Autodesk Inventor part; units mm, degrees
ref_plane "YZ Plane" through (0, 0, 0) normal (1, 0, 0) x (0, 1, 0)
ref_plane "XZ Plane" through (0, 0, 0) normal (0, 1, 0) x (-1, 0, 0)
ref_plane "XY Plane" through (0, 0, 0) normal (0, 0, 1) x (1, 0, 0)
sketch "Sketch1" plane through (0, 0, 0) normal (0, 1, 0) x (-1, 0, 0)
  arc A0 (41.4246, 2.5) -> (41.4246, -2.5) centre (0, 0) ccw construction
  line L0 (0, -41.5) -> (0, 41.5)
  line L1 (0, 0) -> (41.5, 0) construction
  line L2 (41.4246, 2.5) -> (43.7, 2.5)
  line L3 (43.7, 2.5) -> (43.7, -2.5)
  line L4 (43.7, -2.5) -> (41.4246, -2.5)
  line L5 (39.3, 2.5) -> (43.7, -2.5) construction
  line L6 (43.7, 2.5) -> (39.3, -2.5) construction
  arc A1 (0, -41.5) -> (41.4246, -2.5) centre (0, 0) ccw
  arc A2 (41.4246, 2.5) -> (0, 41.5) centre (0, 0) ccw
  line L7 (41.4246, -2.5) -> (41.4246, 2.5) construction
  line L8 (2, 39.4493) -> (2, -39.4493)
  arc A3 (2, -39.4493) -> (39.4968, -0.5) centre (0, 0) ccw
  line L9 (39.4968, -0.5) -> (41.7, -0.5)
  line L10 (41.7, -0.5) -> (41.7, 0.5)
  line L11 (41.7, 0.5) -> (39.4968, 0.5)
  arc A4 (39.4968, 0.5) -> (2, 39.4493) centre (0, 0) ccw
  dimension "d0" = 83
  dimension "d1" = 83
  dimension "d2" = 5
  dimension "d4" = 2.2
  dimension "d5" = 41.5
  dimension "d6" = 2
extrude "Extrusion1" add sketch "Sketch1" against normal blind 2 contours L0 A2 L2 L3 L4 A1 | A4 L11 L10 L9 A3 L8
extrude "Extrusion2" add sketch "Sketch1" along normal blind 173
sketch "Sketch2" plane through (0, -2, 41.5) normal (1, 0, 0) x (0, 0, -1)
  circle A0 centre (12, 12) radius 4.5
  line L0 (83, 0) -> (0, 0)
  line L1 (0, 0) -> (0, 175)
  point P0 (41.5, 2)
  dimension "d11" = 9
  dimension "d12" = 12
  dimension "d13" = 12
extrude "Extrusion3" cut sketch "Sketch2" against normal blind 10
properties part number "_3DPrint"
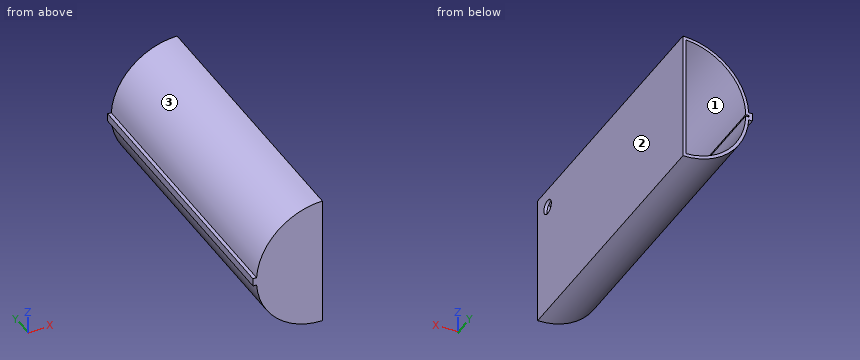
The listing builds one solid part. Answer for the finished solid, in the listing's coordinates (mm). Face numbers are marked on the shaded views. Give positions to 0.01 mm unless a question says otherwise; leave off trailing zeros. Order: outer loops, then holes, each group sorted by start corner. A loop starts at its lowest first (then second) coordinate and runs counter-clockwise, first axis right, second up. Notation, with made-up numbers: (88.25, -33.75) -> (119.25, -33.75) arc R24 cw to (119.25, -10.75) -> close; hole circle Ø2 at (-9, 47). An arc over 180 degrees is marked (long way). Write each question's results on one line, items separated by ' | '.
Q1. Determine the mould class of the marked faces 1, 2 and 3 for opening direction Z: pulls with the +Z half, pulls with the -Z half, needs draft (parallel to the pull), parting line crosses it, or undercut.
Checked values:
face 1: undercut | face 2: needs draft | face 3: pulls with the +Z half
Q2. The part is cut by section A-A, the plane y = 153. Give the vertices of the cut face in (x, z).
Checked values:
outline: (-43.7, -2.5) -> (-41.42, -2.5) arc R41.5 ccw to (0, -41.5) -> (0, 41.5) arc R41.5 ccw to (-41.42, 2.5) -> (-43.7, 2.5) -> close; hole (-41.7, -0.5) -> (-39.5, -0.5) arc R39.5 ccw to (-2, -39.45) -> (-2, 39.45) arc R39.5 ccw to (-39.5, 0.5) -> (-41.7, 0.5) -> close
Q3. The part is cut by section D-D, the plane x = -26.5. Give the vertices of the cut face in (y, z), and give its area (3 significant figures).
Checked values:
outline: (-2, -31.94) -> (173, -31.94) -> (173, -29.29) -> (0, -29.29) -> (0, 29.29) -> (173, 29.29) -> (173, 31.94) -> (-2, 31.94) -> close | area: 1,040 mm^2
Q4. Straight lines are drawn through the part: probe 1 along Y at (x, z) = (-0.55, 29.5); probe 2 along X at (y, z) = (132, -2); probe 3 along X at (y, z) = (139.5, -1.5). For each, find the intervals that lie inside material, in ascending order. Write a range as from..to.
Checked values:
probe 1: y = -2..5.5, 14.5..173 | probe 2: x = -43.7..-39.45, -2..0 | probe 3: x = -43.7..-39.47, -2..0
Q5. Each of these flat-tipped pins is pushed along its axis until it touches: P1, Ø12, axis at x = -14.5, y = 77.5, coming from the +Z side; P2, Ø10, axis at x = -8, y = 125, coming from the -Z side; P3, Ø3, axis at x = -8.5, y = 152.5, coming from the -Z side; P4, Ø10, axis at x = -32.5, z = 18.5, coming from the +Y side. Where does it stop, or does it pass through?
Checked values:
P1: stops at z = 40.62 | P2: stops at z = -41.39 | P3: stops at z = -40.91 | P4: stops at y = 173
Q6. The part is cut by section C-C, the plane y = 10. Give the vertices of the cut face in (x, z), and give its area (3 significant figures).
Checked values:
outline: (-43.7, -2.5) -> (-41.42, -2.5) arc R41.5 ccw to (0, -41.5) -> (0, 25) -> (-2, 25) -> (-2, -39.45) arc R39.5 cw to (-39.5, -0.5) -> (-41.7, -0.5) -> (-41.7, 0.5) -> (-39.5, 0.5) arc R39.5 cw to (-2, 39.45) -> (-2, 34) -> (0, 34) -> (0, 41.5) arc R41.5 ccw to (-41.42, 2.5) -> (-43.7, 2.5) -> close | area: 403 mm^2
Q7. The part is cut by section B-B, the plane z = 31. Give the vertices of the cut face in (x, y).
Checked values:
outline: (-27.59, -2) -> (0, -2) -> (0, 5.76) -> (-2, 5.76) -> (-2, 0) -> (-24.48, 0) -> (-24.48, 173) -> (-27.59, 173) -> close; (-2, 14.24) -> (0, 14.24) -> (0, 173) -> (-2, 173) -> close
